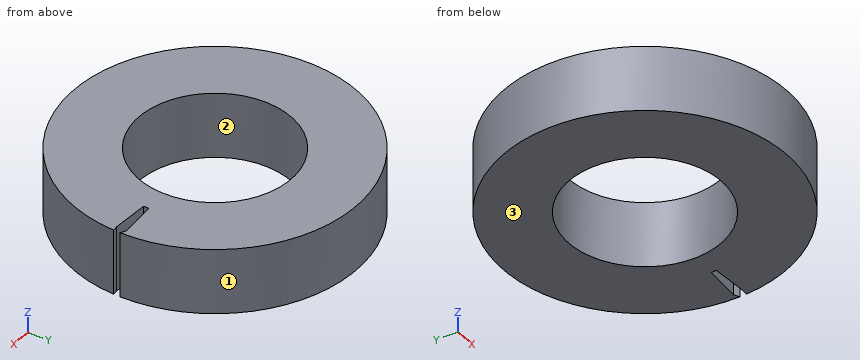
```python
from build123d import *

# Parameters (mm, degrees)
SKETCH_1_R          = 65
SKETCH_1_R_2        = 35
STATOR_BLANK_DEPTH  = 15
SLOT_CUT_TEST_DEPTH = 20


with BuildPart() as part:
    # Эскиз1 → Stator_blank (new, symmetric)
    with BuildSketch(Plane.XY):
        Circle(SKETCH_1_R)
        Circle(SKETCH_1_R_2, mode=Mode.SUBTRACT)
    extrude(amount=STATOR_BLANK_DEPTH, both=True)

    # Эскиз2 → Slot_cut_test (cut, symmetric)
    with BuildSketch(Plane.XY):
        Polygon((46, -1.25), (62.5, -2.25), (67, -1.75), (67, 0), (62.5, 2.25), (46, 1.125), align=None)
    extrude(amount=SLOT_CUT_TEST_DEPTH, both=True, mode=Mode.SUBTRACT)


solid = part.part
```
Could you check a few things on this model? Use its own coordinates, in mm. Face numbers are marked on the shaded views. Round coordinates to 2 decimals unless told otherwise and drop trailing zeros. Order: outer loops, then holes, each group sorted by start corner. A loop starts at its lowest first (then second) coordinate and runs counter-clockwise, first axis right, second up. Notation, with made-up numbers: M -37.75,-7 L 13.25,-7 A16 cw 13.25,8 Z; hole C -16.5,10.5 d4. An arc over 180 degrees is marked long. One line per question, with ' | ' between items. Start each with the question number.
(1) Thinking about a two-plate mould opening in X: for the marked faces 1, 2 and 3, which applies, +X half, -X half, draft (parallel to the pull), parting line (faces both ways), or undercut?
(2) Suppose I cut it at B-B on x = 0. List the corners of the cut face in (y, z) for me, then the cut area to 3 significant figures.
(3) Suppose I cut it at D-D on x = -55. List the corners of the cut face in (y, z) for me, then the cut area to 3 significant figures.
(4) Suppose I cut it at C-C on y = 23. List the corners of the cut face in (x, z) for me.
(5) Please list where these lines run through material, in increasing order: line 1 along Y through (x, z) = (0, 4.5); line 2 along X through (y, z) = (0.5, -12.5); line 3 along Y through (x, z) = (-31, -4).
(6) For P1, Ø10, axis at x = -31, z = -11, coming from the -Y side; P2, Ø5, axis at y = -32.5, z = 4.5, coming from the +X side; P3, Ø2, axis at x = 36.5, z = 10, coming from the +Y side, each with a flat end and sliding along its axis, tell me the tip position at first contact or that it passes through.
(7) Suppose I cut it at A-A on z = 5.5. List the corners of the cut face in (x, y) for me (3 decimals).
Geometry results:
1) face 1: parting line | face 2: undercut | face 3: draft
2) outline: M -65,-15 L -35,-15 L -35,15 L -65,15 Z; M 35,-15 L 65,-15 L 65,15 L 35,15 Z | area: 1,800 mm²
3) outline: M -34.64,-15 L 34.64,-15 L 34.64,15 L -34.64,15 Z | area: 2,080 mm²
4) outline: M -60.79,-15 L -26.38,-15 L -26.38,15 L -60.79,15 Z; M 26.38,-15 L 60.79,-15 L 60.79,15 L 26.38,15 Z
5) line 1: -65 to -35, 35 to 65 | line 2: -65 to -35, 35 to 46 | line 3: -57.13 to -16.25, 16.25 to 57.13
6) P1: y = -59.57 | P2: x = 57.66 | P3: y = 54.45
7) outline: M 46,-1.25 L 46,1.125 L 62.5,2.25 L 64.992,1.004 A65 ccw long 64.97,-1.976 L 62.5,-2.25 Z; hole C 0,0 d70
